Source: CAD feature listing. Evaluate the final solid. Frame: model axes, mm. Face numbers are marked on the shaded views. A direction names the side the tool comes from. Coordinates: 2 decimals unless noted, no trailing zeros. Order: outer loops, then holes, each group sorted by start corner. A loop starts at its lowest first (then second) coordinate and runs counter-clockwise, first axis right, second up. Notation, with made-up numbers: (36.25, -4) - (54.25, -4) arc R20 ccw to (54.25, 22) - close; hole circle Ø10 at (-23, 80). An arc over 180 degrees is marked (long way). One line per question, with ' | ' between items. Start each with the question number.
(1) Draft query along X for the marked faces 1, 2 and 3. Return one class per face: +X half, -X half, draft (parallel to the pull), parting line (faces both ways), or undercut.
(2) Line query: line 1 along Y through (x, z) = (9.5, 0); line 2 along Z through (x, y) = (6, -4); line 3 along X through (y, z) = (3.75, -9) (3 decimals). Output: solid intervals per line, ascending.
(3) Contact query for flat-ended pins moving along their axis: P1, Ø5, axis at x = 34, z = 3.5, coming from the -Y side; P2, Ø4, axis at y = -10.5, z = -5, coming from the +X side (3 decimals); P3, Ø1.5, axis at y = 0, z = 1.5, coming from the -X side. Output: stop coordinate, or through.
(4) Section B-B (x = 8). Return the cut outline in (y, z) (1 decimal), then the cut area to 3 significant figures.
(5) Section A-A (x = 4). Return the cut outline in (y, z) (1 decimal), then the cut area to 4 significant figures.
(6) Access query for the marked faces 4, 5 and 6. Directions: +Z, -Z, +X, -X, +Y, -Y. A direction counts if a zero-diameter tool reaches every point of the face in a straight line with its end or side. Return the directions, or none.
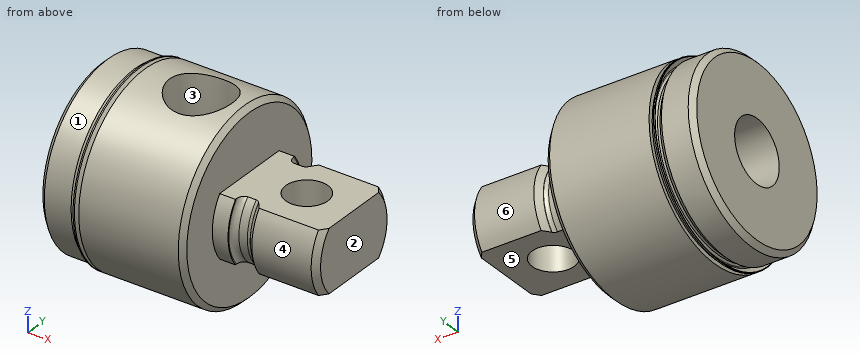
from build123d import *

# Parameters (mm, degrees)
SKETCH3_W               = 56.4388
SKETCH3_H               = 112.8776
SKETCH3_W_2             = 9.4615
SKETCH3_H_2             = 56.4388
CUT_EXTRUDE1_DEPTH      = 15.875
HOLE1_D                 = 9.525
HOLE1_DEPTH             = 20.955
HOLE1_TIP               = 2.749630657
SKETCH8_R               = 3.2004
CUT_EXTRUDE2_DEPTH      = 7.096125
CUT_EXTRUDE2_DEPTH_BACK = 7.096125


with BuildPart() as part:
    # Sketch1 → Revolve1 (revolve)
    with BuildSketch(Plane.XY):
        Polygon((0, 0), (0, 12.84605), (0.762, 13.60805), (4.826, 13.60805), (5.588, 12.84605), (6.35, 12.84605), (6.35, 14.1097), (21.463, 14.1097), (22.225, 13.3477), (22.225, 0), align=None)
    revolve(axis=Axis((22.225, 0, 0), (-1, 0, 0)))

    # Sketch2 → Revolve2 (revolve)
    with BuildSketch(Plane.XY):
        with BuildLine():
            Line((22.225, 0), (22.225, 7.90575))
            Line((22.225, 7.90575), (24.6126, 7.90575))
            Line((24.6126, 7.90575), (24.6126, 7.72795))
            ThreePointArc((24.6126, 7.72795), (24.872982072, 7.099332072), (25.5016, 6.83895))
            Line((25.5016, 6.83895), (26.7843, 6.83895))
            ThreePointArc((26.7843, 6.83895), (27.10530348, 6.898927826), (27.38299292, 7.0707683))
            Line((27.38299292, 7.0707683), (27.412917928, 7.09803))
            Line((27.412917928, 7.09803), (28.252387928, 7.9375))
            Line((28.252387928, 7.9375), (37.26053, 7.9375))
            Line((37.26053, 7.9375), (38.1, 7.09803))
            Line((38.1, 7.09803), (38.1, 0))
            Line((38.1, 0), (22.225, 0))
        make_face()
    revolve(axis=Axis((38.1, 0, 0), (-1, 0, 0)))

    # Sketch3 → Cut-Extrude1 (cut)
    with BuildSketch(Plane(origin=(38.1, 0, 0), x_dir=(0, 0, -1), z_dir=(1, 0, 0))):
        Rectangle(SKETCH3_W, SKETCH3_H)
        Rectangle(SKETCH3_W_2, SKETCH3_H_2, mode=Mode.SUBTRACT)
    extrude(amount=-CUT_EXTRUDE1_DEPTH, mode=Mode.SUBTRACT)

    # Hole1
    with Locations(Plane.ZY):
        with Locations((0, 0)):
            Hole(HOLE1_D / 2, depth=HOLE1_DEPTH)
            with Locations((0, 0, -(HOLE1_DEPTH + HOLE1_TIP / 2))):  # 120° drill point
                Cone(0, HOLE1_D / 2, HOLE1_TIP, mode=Mode.SUBTRACT)

    # Sketch6 → Cut-Revolve1 (revolve, cut)
    with BuildSketch(Plane(origin=(0, 0, 0), x_dir=(1, 0, 0), z_dir=(0, 0.999847695, 0.017452406))):
        Polygon((15.0876, 0), (19.710593378, 0), (19.710593378, -7.1755), (19.927075925, -14.1097), (15.0876, -14.1097), align=None)
    revolve(axis=Axis((15.0876, -0.246248219, 14.107551024), (0, 0.017452406, -0.999847695)), mode=Mode.SUBTRACT)

    # Sketch7 → Revolve3 (revolve)
    with BuildSketch(Plane.XY):
        with BuildLine():
            Line((5.48614893, 14.025531804), (6.227512806, 13.284167928))
            ThreePointArc((6.227512806, 13.284167928), (6.264710245, 13.194365367), (6.227512806, 13.104562806))
            Line((6.227512806, 13.104562806), (5.969, 12.84605))
            Line((5.969, 12.84605), (5.588, 12.84605))
            Line((5.588, 12.84605), (5.588, 12.59205))
            Line((5.588, 12.59205), (6.35, 12.59205))
            Line((6.35, 12.59205), (6.35, 13.44904893))
            Line((6.35, 13.44904893), (5.68934893, 14.1097))
            Line((5.68934893, 14.1097), (5.48614893, 14.1097))
            Line((5.48614893, 14.1097), (5.48614893, 14.025531804))
        make_face()
    revolve(axis=Axis((6.35, 0, 0), (-1, 0, 0)))

    # Sketch8 → Cut-Extrude2 (cut, two sides)
    with BuildSketch(Plane.XY) as cut_extrude2_sk:
        with Locations((30.9626, 0)):
            Circle(SKETCH8_R)
    extrude(amount=CUT_EXTRUDE2_DEPTH, mode=Mode.SUBTRACT)
    extrude(cut_extrude2_sk.sketch, amount=-CUT_EXTRUDE2_DEPTH_BACK, mode=Mode.SUBTRACT)


solid = part.part
Response values:
1) face 1: draft | face 2: +X half | face 3: undercut
2) line 1: y = -14.11 to -4.76, 4.76 to 14.11 | line 2: z = -13.21 to -12.91, -12.24 to -2.58, 2.58 to 12.24, 12.91 to 13.21 | line 3: x = 0 to 22.225
3) P1: stops at y = -7.87 | P2: stops at x = 22.225 | P3: stops at x = 22.41
4) outline: circle Ø28.2 at (0, 0); hole circle Ø9.5 at (0, 0) | area: 554 mm²
5) outline: circle Ø27.2 at (0, 0); hole circle Ø9.5 at (0, 0) | area: 510.5 mm²
6) face 4: +X, -Y | face 5: -Z, +X, +Y, -Y | face 6: +X, +Y
